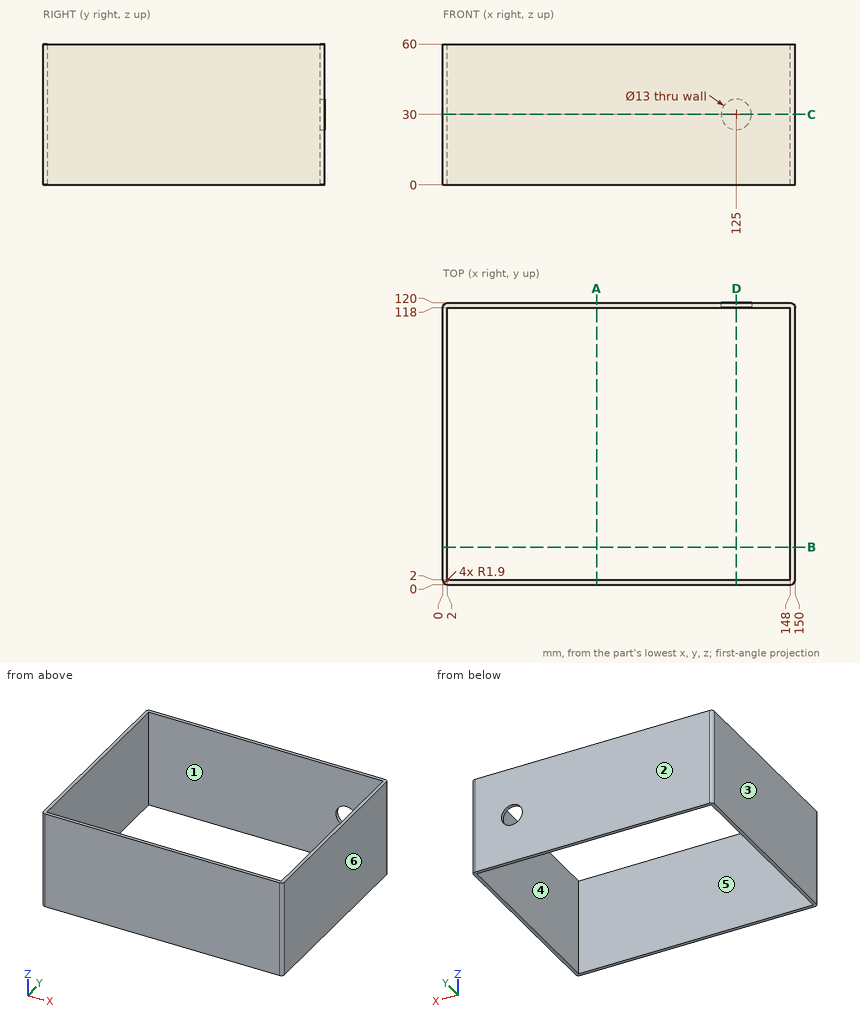
Can you work these out from the drawing? Everything is in mm from the part's minimum corner. A direction names the side the tool comes from. Round coordinates to 2 decimals unless told otherwise and drop trailing zeros. Loops run counter-clockwise (first coordinate to the right, second up) from the corner with the lowest first, then second, coordinate; pieces in that order, holes last.
1. If we section it at A-A on x = 65.5: Write out the boundary of the cut face in (y, z).
Answer list:
outline: (0, 0) - (2, 0) - (2, 60) - (0, 60) - close; (118, 0) - (120, 0) - (120, 60) - (118, 60) - close
2. If I drill on line 1 along Y through (x, z) = (71.5, 12); line 2 along X through (y, z) = (76.5, 13); line 3 along Z through (x, y) = (125, 119.45), over which ranges is the centre line in solid material (lowest first)?
Answer list:
line 1: y = 0 to 2, 118 to 120
line 2: x = 0 to 2, 148 to 150
line 3: z = 0 to 23.5, 36.5 to 60
3. We'd pull the mould along X, two halves only. Please class the marked faces 1, 2, 3 and 4: +X half, -X half, draft (parallel to the pull), parting line (faces both ways), or undercut.
Answer list:
face 1: undercut
face 2: draft
face 3: -X half
face 4: undercut
4. If we section it at C-C on z = 30: Write out the boundary of the cut face in (x, y), plus the area to 3 significant figures.
Answer list:
outline: (0, 1.9) arc R1.9 ccw to (1.9, 0) - (148.1, 0) arc R1.9 ccw to (150, 1.9) - (150, 118.1) arc R1.9 ccw to (148.1, 120) - (131.5, 120) - (131.5, 118) - (148, 118) - (148, 2) - (2, 2) - (2, 118) - (118.5, 118) - (118.5, 120) - (1.9, 120) arc R1.9 ccw to (0, 118.1) - close
area: 1,030 mm2
5. Which directions (+Z, -Z, +X, -X, +Y, -Y) give clear straight access to the entire face, cutting with the end or side of a thin tool? Please do the marked faces 5 and 6.
Answer list:
face 5: +Z, -Z
face 6: +Z, -Z, +X, +Y, -Y
6. If we section it at B-B on y = 16: Write out the boundary of the cut face in (x, z), plus the area to 3 significant figures.
Answer list:
outline: (0, 0) - (2, 0) - (2, 60) - (0, 60) - close; (148, 0) - (150, 0) - (150, 60) - (148, 60) - close
area: 240 mm2
7. If we section it at D-D on x = 125: Write out the boundary of the cut face in (y, z).
Answer list:
outline: (0, 0) - (2, 0) - (2, 60) - (0, 60) - close; (118, 0) - (120, 0) - (120, 23.5) - (118, 23.5) - close; (118, 36.5) - (120, 36.5) - (120, 60) - (118, 60) - close
